Work out the finished part from the listing and answer in its coordinate system (mm). Face numbers are marked on the shaded views. A direction names the side the tool comes from. Round coordinates to 2 decimals unless told otherwise and drop trailing zeros. Loops run counter-clockwise (first coordinate to the right, second up) from the corner with the lowest first, then second, coordinate; pieces in that order, holes last. Notation, with made-up numbers: M -23,23.5 L -2,23.5 A26 ccw -2,37.5 Z; hole C 63,74.25 d9. An arc over 180 degrees is marked long. One line per item, written item: value.
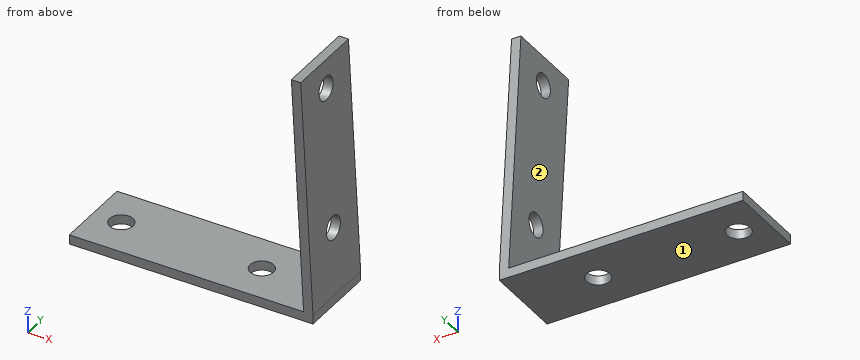
```python
from build123d import *

# Parameters (mm, degrees)
ESQUISSE1_W             = 52
ESQUISSE1_H             = 17
BOSS_EXTRU_1_DEPTH      = 2
ESQUISSE2_W             = 2
ESQUISSE2_H             = 17
BOSS_EXTRU_2_DEPTH      = 50
ESQUISSE3_R             = 2.5
ENL_V_MAT_EXTRU_1_DEPTH = 50
ESQUISSE4_R             = 2.5
ENL_V_MAT_EXTRU_2_DEPTH = 50


with BuildPart() as part:
    # Esquisse1 → Boss.-Extru.1 (new body)
    with BuildSketch(Plane.XY):
        Rectangle(ESQUISSE1_W, ESQUISSE1_H)
    extrude(amount=BOSS_EXTRU_1_DEPTH)

    # Esquisse2 → Boss.-Extru.2 (add, along a direction that is not the sketch's normal)
    with BuildSketch(Plane.XY.offset(2)):
        with Locations((25, 0)):
            Rectangle(ESQUISSE2_W, ESQUISSE2_H)
    extrude(amount=BOSS_EXTRU_2_DEPTH, dir=(-0.052335956242937125, 0, 0.9986295347545743))

    # Esquisse3 → Enlèv. mat.-Extru.1 (cut)
    with BuildSketch(Plane.XY.offset(2)):
        with Locations((-20, 0)):
            Circle(ESQUISSE3_R)
        with Locations((10, 0)):
            Circle(ESQUISSE3_R)
    extrude(amount=-ENL_V_MAT_EXTRU_1_DEPTH, mode=Mode.SUBTRACT)

    # Esquisse4 → Enlèv. mat.-Extru.2 (cut)
    with BuildSketch(Plane(origin=(24.038791208, 0, 1.259819664), x_dir=(-0.052335956242937125, 0, 0.9986295347545743), z_dir=(-0.9986295347545743, 0, -0.052335956242937125))):
        with Locations((44.74119612, 0)):
            Circle(ESQUISSE4_R)
        with Locations((14.74119612, 0)):
            Circle(ESQUISSE4_R)
    extrude(amount=-ENL_V_MAT_EXTRU_2_DEPTH, mode=Mode.SUBTRACT)


solid = part.part
```
1) Find section C-C (y = 5.25). Give the vertices of the cut face in (x, z), then the cut area to 3 significant figures.
Check values:
outline: M -26,0 L 26,0 L 26,2 L 23.38,51.93 L 21.38,51.93 L 24,2 L -26,2 Z
area: 204 mm2
2) Find section B-B (y = 0). Give the vertices of the cut face in (x, z).
Check values:
outline: M -26,0 L -22.5,0 L -22.5,2 L -26,2 Z; M -17.5,0 L 7.5,0 L 7.5,2 L -17.5,2 Z; M 12.5,0 L 26,0 L 26,2 L 25.39,13.59 L 23.4,13.48 L 24,2 L 12.5,2 Z; M 21.38,51.93 L 21.57,48.44 L 23.56,48.54 L 23.38,51.93 Z; M 21.83,43.44 L 23.14,18.48 L 25.13,18.58 L 23.82,43.55 Z
3) Find section D-D (x = 19.5). Give the vertices of the cut face in (y, z), then the cut area to 3 significant figures.
Check values:
outline: M -8.5,0 L 8.5,0 L 8.5,2 L -8.5,2 Z
area: 34.0 mm2
4) Find the intervals of material crossed by probe 1 along Y at (x, z) = (-20, 1.35); probe 2 along Z at (x, y) = (-14, 5.25); probe 3 along X at (y, z) = (-6.5, 6.5), in increasing order. Write a range as from..to.
Check values:
probe 1: -8.5..-2.5, 2.5..8.5
probe 2: 0..2
probe 3: 23.76..25.76
5) Find section A-A (x = -20). Give the vertices of the cut face in (y, z), then the cut area to 3 significant figures.
Check values:
outline: M -8.5,0 L -2.5,0 L -2.5,2 L -8.5,2 Z; M 2.5,0 L 8.5,0 L 8.5,2 L 2.5,2 Z
area: 24.0 mm2
6) Each of these flat-tipped pins is pushed along its axis until it touches: pin 1 (2 mm diameter, centred on y = -5.5, z = 7, fed in from +X); pin 2 (6 mm diameter, centred on x = -20, y = 0, fed in from +Z); pin 3 (2 mm diameter, centred on y = -4.5, z = 32, fed in from -X). Where does it stop, or does it pass through?
Check values:
pin 1: x = 25.79
pin 2: z = 2
pin 3: x = 22.38
7) For the marked faces 1 and 2, determine the directions among +Z, -Z, +X, -X, +Y, -Y from which every point of the face is accessible in a straight line to the end or side of a thin tool.
Check values:
face 1: -Z, +X, -X, +Y, -Y
face 2: -X, +Y, -Y
